Geometry: final body of the model. Coordinates: model frame, mm. Face numbers are marked on the shaded views. Give positions to 0.01 mm unless a question says otherwise; leave off trailing zeros. Write each loop counter-clockwise with the first axis right and the second up, starting at its lowest first coordinate (ties: lowest second). Pieces come first, ordered by that corner, then holes.
Q1. Line query: L1, parallel to X at y = -4, z = -1.5; L2, parallel to Z at x = 4.5, y = -7; L3, parallel to Y at x = -73.5, z = -9. Output: solid intervals per line, ascending.
Q2. Cut plane A-A on y = -4.25. Return the cut outline in (x, z).
Q3. Draft query along Z for the marked faces 1, 2 and 3. Return one class per face: pulls with the +Z half, pulls with the -Z half, needs draft (parallel to the pull), parting line crosses it, or undercut.
Q4. Cut plane C-C on x = 18. Return the cut outline in (y, z).
Q5. Cut plane B-B on z = -8. Return the cut outline in (x, y).
Q6. Cut plane D-D on z = 13. Return the cut outline in (x, y).
Q7. Pin query (flat end, axial travel): pin 1 (2 mm diameter, centred on x = 13.5, y = -3.5, fed in from -Z); pin 2 (12 mm diameter, centred on y = -6.5, z = 11, fed in from +X); pin 3 (5 mm diameter, centred on x = 57, y = -3.5, fed in from -Z). Return the tip coordinate at first contact, or that it passes through.
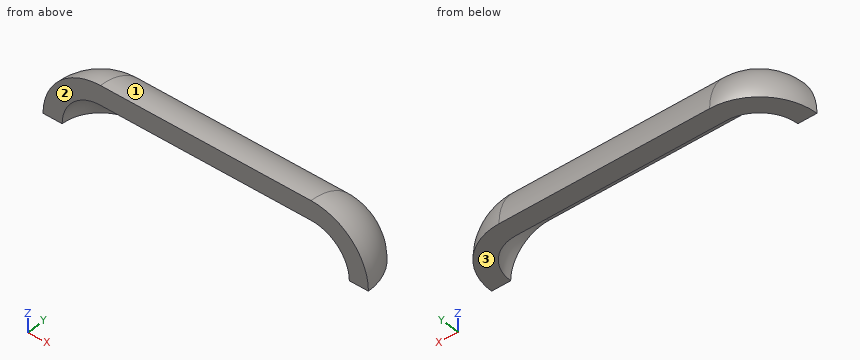
Autodesk Inventor part; units mm, degrees
sketch "Эскиз3" plane through (0, 0, 0) normal (1, 0, 0) x (0, 1, 0)
  line L0 (-10.6066, -10.6066) -> (-10.6066, 19.3934)
  line L1 (-10.6066, -10.6066) -> (19.3934, -10.6066)
  arc A0 (19.3934, -10.6066) -> (-10.6066, 19.3934) centre (-10.6066, -10.6066) ccw
  line L2 (-10.6066, -10.6066) -> (10.6066, 10.6066) construction
  point P0 (0, 0)
  point P1 (0, 0)
  dimension "d9" = 30
extrude "Выдавливание3" add sketch "Эскиз3" along normal mid plane 110
sketch "Эскиз4" plane through (55, 0, 0) normal (1, 0, 0) x (0, 0, -1)
  line L0 (-19.3934, -10.6066) -> (10.6066, -10.6066)
  line L1 (10.6066, -10.6066) -> (10.6066, 19.3934)
  arc A0 (10.6066, 19.3934) -> (-19.3934, -10.6066) centre (10.6066, -10.6066) ccw
  point P0 (0, 0)
revolve "Вращение1" add sketch "Эскиз4" angle 90 about axis through (55, -10.6066, -10.6066) along (0, 1, 0)
mirror "Зеркальное отражение1" about plane through (0, 0, 0) normal (1, 0, 0) of "Вращение1"
shell "Оболочка2" thickness 10 removed faces 2 at (18.3333, -10.6066, -0.6066) at (18.3333, -0.6066, -10.6066)
properties part number "Козырёк_для_камеры"
Data:
1. L1: x = -82.81 to -71.54, 71.54 to 82.81
1. L2: z = 9.07 to 19.18
1. L3: y = -3.18 to 12.96
2. outline: (-84.32, -10.61) - (-73.96, -10.61) arc R18.96 cw to (-55, 8.36) - (55, 8.36) arc R18.96 cw to (73.96, -10.61) - (84.32, -10.61) arc R29.32 ccw to (55, 18.71) - (-55, 18.71) arc R29.32 ccw to start
3. face 1: pulls with the +Z half
3. face 2: needs draft
3. face 3: pulls with the -Z half
4. outline: (-10.61, 9.39) arc R20 cw to (9.39, -10.61) - (19.39, -10.61) arc R30 ccw to (-10.61, 19.39) - close
5. outline: (-84.89, -10.61) - (-74.83, -10.61) arc R19.83 cw to (-55, 9.22) - (55, 9.22) arc R19.83 cw to (74.83, -10.61) - (84.89, -10.61) arc R29.89 ccw to (55, 19.28) - (-55, 19.28) arc R29.89 ccw to start
6. outline: (-73.51, -10.61) - (73.51, -10.61) arc R18.51 ccw to (55, 7.91) - (-55, 7.91) arc R18.51 ccw to start
7. pin 1: stops at z = 7.68
7. pin 2: stops at x = 80.38
7. pin 3: stops at z = 6.78
